```python
from build123d import *

# Parameters (mm, degrees)
SKETCH_1_R                   = 29.5
EXTRUDE_1_DEPTH              = 3
HOLE_WIZARD_M3_1_D           = 2.5
HOLE_WIZARD_M3_1_CSINK_D     = 2.55
HOLE_WIZARD_M3_1_CSINK_ANGLE = 90
HOLE_WIZARD_M3_2_D           = 2.5
HOLE_WIZARD_M3_2_CSINK_D     = 2.55
HOLE_WIZARD_M3_2_CSINK_ANGLE = 90


with BuildPart() as part:
    # 草图1 → 凸台-拉伸1 (new body)
    with BuildSketch(Plane(origin=(0, 0, 0), x_dir=(1, 0, 0), z_dir=(0, 1, 0))):
        Circle(SKETCH_1_R)
    extrude(amount=EXTRUDE_1_DEPTH)

    # M3 螺纹孔的螺纹孔钻头1 (through all)
    with Locations(Plane(origin=(0, 3, 0), x_dir=(1, 0, 0), z_dir=(0, 1, 0))):
        with Locations((6.180339887, 19.021130326), (20, 0), (6.180339887, -19.021130326), (-16.180339887, -11.755705046), (-16.180339887, 11.755705046)):
            CounterSinkHole(HOLE_WIZARD_M3_1_D / 2, HOLE_WIZARD_M3_1_CSINK_D / 2, counter_sink_angle=HOLE_WIZARD_M3_1_CSINK_ANGLE)

    # M3 螺纹孔的螺纹孔钻头2 (through all)
    with Locations(Plane(origin=(0, 3, 0), x_dir=(1, 0, 0), z_dir=(0, 1, 0))):
        with Locations((0, 0), (7.071067812, 0), (0, -7.071067812), (-7.071067812, 0), (0, 7.071067812)):
            CounterSinkHole(HOLE_WIZARD_M3_2_D / 2, HOLE_WIZARD_M3_2_CSINK_D / 2, counter_sink_angle=HOLE_WIZARD_M3_2_CSINK_ANGLE)


solid = part.part
```
Verification items for the finished model (mm, model axes). Round coordinates to 2 decimals unless told otherwise and drop trailing zeros. Write each loop counter-clockwise with the first axis right and the second up, starting at its lowest first coordinate (ties: lowest second). Pieces come first, ordered by that corner, then holes.
1. Draft check along Z on faces 1 (the cylindrical face through (18.845, 1.467, 0.479)), 2 (the cylindrical face through (28.14, 1.48, -8.86)), 3 (the flat face through (6, 3, 6)). Enter one of: +Z half, -Z half, draft (parallel to the pull), parting line (faces both ways), or undercut.
2. Section check B-B on x = 0. Enter the section's corners in (y, z) (3 decimals), plus the area to 3 significant figures.
3. Section check D-D on x = 20. Enter the section's corners in (y, z) (3 decimals).
4. Scan lines: L1, parallel to Z at x = 0, y = 2.2; L2, parallel to X at y = 0.2, z = -1; L3, parallel to Z at x = -17, y = 0.75. Record each from-to range of solid material in increasing order.
5. Section check A-A on z = 0. Enter the section's corners in (x, y) (3 decimals).
6. Section check C-C on y = 1.2. State how many separate pieces and enclosed holes the cut face has, plus the area to 3 significant figures.
7. Gauge pin test, flat ends, axial feed: P1, Ø1.5, axis at x = 0, z = 7.07, coming from the -Y side; P2, Ø1, axis at y = 2, z = 6.5, coming from the +X side. Record the tip position at first contact, or that the pin passes through.
Answer:
1. face 1: undercut
1. face 2: parting line
1. face 3: draft
2. outline: (0, -29.5) - (3, -29.5) - (3, -8.346) - (2.975, -8.321) - (0, -8.321) - close; (0, -5.821) - (2.975, -5.821) - (3, -5.796) - (3, -1.275) - (2.975, -1.25) - (0, -1.25) - close; (0, 1.25) - (2.975, 1.25) - (3, 1.275) - (3, 5.796) - (2.975, 5.821) - (0, 5.821) - close; (0, 8.321) - (2.975, 8.321) - (3, 8.346) - (3, 29.5) - (0, 29.5) - close
2. area: 154 mm2
3. outline: (0, -21.685) - (3, -21.685) - (3, -1.275) - (2.975, -1.25) - (0, -1.25) - close; (0, 1.25) - (2.975, 1.25) - (3, 1.275) - (3, 21.685) - (0, 21.685) - close
4. L1: z = -29.5 to -8.32, -5.82 to -1.25, 1.25 to 5.82, 8.32 to 29.5
4. L2: x = -29.48 to -7.82, -6.32 to -0.75, 0.75 to 6.32, 7.82 to 19.25, 20.75 to 29.48
4. L3: z = -24.11 to -12.7, -10.81 to 10.81, 12.7 to 24.11
5. outline: (-29.5, 0) - (-8.321, 0) - (-8.321, 2.975) - (-8.346, 3) - (-29.5, 3) - close; (-5.821, 0) - (-1.25, 0) - (-1.25, 2.975) - (-1.275, 3) - (-5.796, 3) - (-5.821, 2.975) - close; (1.25, 0) - (5.821, 0) - (5.821, 2.975) - (5.796, 3) - (1.275, 3) - (1.25, 2.975) - close; (8.321, 0) - (18.75, 0) - (18.75, 2.975) - (18.725, 3) - (8.346, 3) - (8.321, 2.975) - close; (21.25, 0) - (29.5, 0) - (29.5, 3) - (21.275, 3) - (21.25, 2.975) - close
6. separate pieces: 1
6. enclosed holes: 10
6. area: 2,680 mm2
7. P1: passes through
7. P2: stops at x = 28.88
